CAD build for the part. Positions are in the model's coordinates, mm. A direction names the side the tool comes from. Coordinates: 2 decimals unless noted, no trailing zeros. Loops run counter-clockwise (first coordinate to the right, second up) from the corner with the lowest first, then second, coordinate; pieces in that order, holes last.
1) Which spindle directions (+Z, -Z, +X, -X, +Y, -Y) get a long thin tool onto all of the face, cutting with end or side? Do faces 4 (the cylindrical face through (14.671, -27.434, 3.431)), 5 (the cylindrical face through (43.9, -18.3, 3.4)). Say none if no direction does.
2) Two-plate mould, pull along X, no slides. Class faces 1 (the cylindrical face through (0.08, 48.49, 3.43)), 2 (the cylindrical face through (-1.4, 41.9, 3.4)), 3 (the flat face through (6, -10, 0)): +X half, -X half, draft (parallel to the pull), parting line (faces both ways), or undercut.
3) Saw through at A-A, the plane y = -2. Write the cut outline in (x, z).
4) Saw through at D-D, the plane y = 36. Write the cut outline in (x, z).
5) Pin check, flat tips, straight feed: pin 1 Ø20 at (x, y) = (0, 30.99) entering from -Z; pin 2 Ø1 at (y, z) = (-24.5, 5) entering from +X; pin 3 Ø2 at (y, z) = (-17.5, 3) entering from -X. Stop position of each tip, or through.
6) Saw through at C-C, the plane z = 1. Write the cut outline in (x, y).
7) Wall check: line 1 along Y through (x, z) = (0, 4.25); line 2 along X through (y, z) = (-20.5, 6.25); line 3 along Y through (x, z) = (9.5, 0.5). Give the ranges that are in metal, low to high.
8) Saw through at B-B, the plane x = 0. Write the cut outline in (y, z).
```python
from build123d import *

# Parameters (mm, degrees)
F0_R     = 11
F1_DEPTH = 6.96


with BuildPart() as f1:
    # F0 (on Top) → F1 (new body)
    with BuildSketch(Plane.XY):
        with BuildLine():
            ThreePointArc((20.967224, 1.44653), (13.484367, 9.343679), (13.791942, 20.218582))
            ThreePointArc((13.791942, 20.218582), (-0.473405, 48.484008), (-13.189176, 19.488428))
            ThreePointArc((-13.189176, 19.488428), (-13.229135, 8.590307), (-21.602449, 1.614759))
            ThreePointArc((-21.602449, 1.614759), (-43.793526, -18.199862), (-16.173887, -29.255114))
            ThreePointArc((-16.173887, -29.255114), (-14.55487, -27.485928), (-12.744492, -25.913108))
            ThreePointArc((-12.744492, -25.913108), (0.13651, -21.532556), (12.995613, -25.976982))
            ThreePointArc((12.995613, -25.976982), (14.693213, -27.456193), (16.222473, -29.108848))
            ThreePointArc((16.222473, -29.108848), (43.988926, -17.774444), (20.967224, 1.44653))
        make_face()
        with Locations((-26.838484, -15.495206)):
            Circle(F0_R, mode=Mode.SUBTRACT)
        Circle(F0_R, mode=Mode.SUBTRACT)
        with Locations((26.838484, -15.495206)):
            Circle(F0_R, mode=Mode.SUBTRACT)
        with Locations((0, 30.990412)):
            Circle(F0_R, mode=Mode.SUBTRACT)
    extrude(amount=F1_DEPTH)


solid = f1.part
```
Data:
1. face 4: +Z, -Z, -Y
1. face 5: +Z, -Z
2. face 1: parting line
2. face 2: undercut
2. face 3: draft
3. outline: (-38.08, 0) - (-10.82, 0) - (-10.82, 6.96) - (-38.08, 6.96) - close; (10.82, 0) - (38.31, 0) - (38.31, 6.96) - (10.82, 6.96) - close
4. outline: (-16.77, 0) - (-9.79, 0) - (-9.79, 6.96) - (-16.77, 6.96) - close; (9.79, 0) - (16.77, 0) - (16.77, 6.96) - (9.79, 6.96) - close
5. pin 1: passes through
5. pin 2: stops at x = 41.76
5. pin 3: stops at x = -44.01
6. outline: (-21.6, 1.61) arc R17.5 ccw (long way) to (-16.17, -29.26) arc R20.98 cw to (-12.74, -25.91) arc R20.98 cw to (13, -25.98) arc R20.98 cw to (16.22, -29.11) arc R17.5 ccw (long way) to (20.97, 1.45) arc R14.19 cw to (13.79, 20.22) arc R17.5 ccw (long way) to (-13.19, 19.49) arc R12.9 cw to start; hole circle Ø22 at (-26.84, -15.5); hole circle Ø22 at (0, 0); hole circle Ø22 at (0, 30.99); hole circle Ø22 at (26.84, -15.5)
7. line 1: y = -21.53 to -11, 11 to 19.99, 41.99 to 48.49
7. line 2: x = -43.23 to -36.63, -17.04 to 17.04, 36.63 to 43.34
7. line 3: y = -23.76 to -5.55, 5.55 to 25.45, 36.54 to 45.69
8. outline: (-21.53, 0) - (-11, 0) - (-11, 6.96) - (-21.53, 6.96) - close; (11, 0) - (19.99, 0) - (19.99, 6.96) - (11, 6.96) - close; (41.99, 0) - (48.49, 0) - (48.49, 6.96) - (41.99, 6.96) - close
